Check sheet for the modelled part. Datum: model origin and axes. Units: mm. Face numbers are marked on the shaded views. Give positions to 0.01 mm unless a question says otherwise; leave off trailing zeros. Write each loop counter-clockwise with the first axis right and the second up, starting at its lowest first coordinate (ties: lowest second). Pieces come first, ordered by that corner, then holes. Notation, with made-up numbers: (69, -1) -> (86, -1) arc R21 ccw to (86, 9) -> close; hole circle Ø8 at (2, 72.25). An arc over 180 degrees is marked (long way). Return JSON: item names as keys, results as strings.
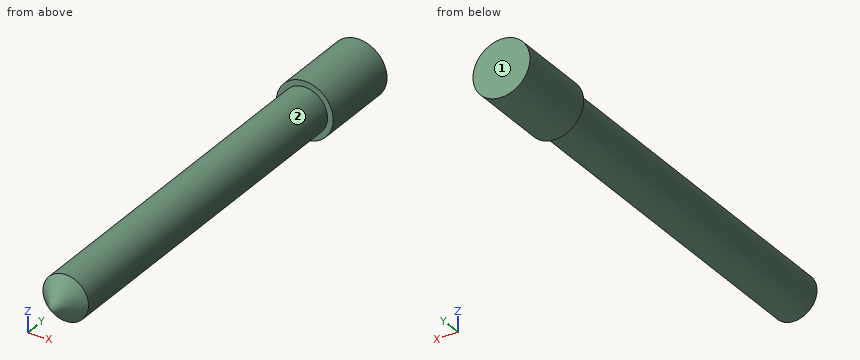
from build123d import *

# Parameters (mm, degrees)
SKETCH1_R           = 5
BOSS_EXTRUDE1_DEPTH = 85
CHAMFER1_SIZE       = 5
SKETCH2_R           = 6.25
BOSS_EXTRUDE2_DEPTH = 18


with BuildPart() as part:
    # Sketch1 → Boss-Extrude1 (new body)
    with BuildSketch(Plane(origin=(0, 0, 0), x_dir=(1, 0, 0), z_dir=(0, 1, 0))):
        Circle(SKETCH1_R)
    extrude(amount=BOSS_EXTRUDE1_DEPTH)

    # Chamfer1
    chamfer1_edges = [part.edges().sort_by_distance(p)[0] for p in [
        (-5, 0, 0),
    ]]
    chamfer(chamfer1_edges, length=CHAMFER1_SIZE)

    # Sketch2 → Boss-Extrude2 (add)
    with BuildSketch(Plane(origin=(0, 85, 0), x_dir=(1, 0, 0), z_dir=(0, 1, 0))):
        Circle(SKETCH2_R)
    extrude(amount=BOSS_EXTRUDE2_DEPTH)


solid = part.part
(1) Release check for a two-part mould opening along X. For the marked faces 1 and 2 record: pulls with the +X half, pulls with the -X half, needs draft (parallel to the pull), parting line crosses it, or undercut.
Reply:
{"face 1": "needs draft", "face 2": "parting line crosses it"}
(2) Thickness scan on L1, parallel to Y at x = 5.75, z = 1.75; L2, parallel to Z at x = -0.25, y = 75; L3, parallel to X at y = 86.5, z = 0.5. Record the ranges inside material, lowest first.
Reply:
{"L1": "85 to 103", "L2": "-4.99 to 4.99", "L3": "-6.23 to 6.23"}
(3) Depth check by flat-ended pin: pin 1 Ø6 at (x, y) = (3.5, 90) entering from +Z; pin 2 Ø1 at (x, z) = (-1.5, -1.5) entering from -Y; pin 3 Ø4 at (x, z) = (-2.5, 1) entering from -Y. Enter the tip coordinate at first touch or a pass-through.
Reply:
{"pin 1": "z = 6.23", "pin 2": "y = 1.62", "pin 3": "y = 0.69"}
(4) Cross-section at B-B on y = 44.5. Enter the section's corners in (x, z).
Reply:
{"outline": "circle Ø10 at (0, 0)"}
(5) Cross-section at A-A on y = 94. Enter the section's corners in (x, z).
Reply:
{"outline": "circle Ø12.5 at (0, 0)"}
